```python
from build123d import *

# Parameters (mm, degrees)
SCHIZZO1_W                   = 120
SCHIZZO1_H                   = 40
ESTRUSIONE_ESTRUSIONE1_DEPTH = 3
SCHIZZO2_R                   = 2.5
TAGLIO_ESTRUSIONE1_DEPTH     = 3
SCHIZZO3_R                   = 2.5
TAGLIO_ESTRUSIONE2_DEPTH     = 3


with BuildPart() as part:
    # Schizzo1 → Estrusione-Estrusione1 (new body)
    with BuildSketch(Plane.XY):
        with Locations((60, -20)):
            Rectangle(SCHIZZO1_W, SCHIZZO1_H)
    extrude(amount=ESTRUSIONE_ESTRUSIONE1_DEPTH)

    # Schizzo2 → Taglio-Estrusione1 (cut)
    with BuildSketch(Plane.XY.offset(3)):
        with Locations((18, -20)):
            Circle(SCHIZZO2_R)
    extrude(amount=-TAGLIO_ESTRUSIONE1_DEPTH, mode=Mode.SUBTRACT)

    # Schizzo3 → Taglio-Estrusione2 (cut)
    with BuildSketch(Plane.XY.offset(3)):
        with Locations((100, -20)):
            Circle(SCHIZZO3_R)
    extrude(amount=-TAGLIO_ESTRUSIONE2_DEPTH, mode=Mode.SUBTRACT)


solid = part.part
```
Input: part model. Units: mm. Frame: model coordinates. Coordinates: 2 decimals unless noted, no trailing zeros. Loops run counter-clockwise (first coordinate to the right, second up) from the corner with the lowest first, then second, coordinate; pieces in that order, holes last. Notation, with made-up numbers: M 88,65.25 L 120,65.25 A18 ccw 120,77.25 Z; hole C 56,69 d6. An arc over 180 degrees is marked long. Use a Markdown table: item, result. Add a question column.
1) Line query: L1, parallel to Y at x = 100, z = 1.7; L2, parallel to X at y = -21, z = 1.35; L3, parallel to Y at x = 20, z = 0.9. Output: solid intervals per line, ascending. Write a range as from..to.
2) Section B-B, the plane x = 100. Return the cut outline in (y, z), plus the area to 3 significant figures.
3) Section A-A, the plane y = -20. Return the cut outline in (x, z).
4) Pin query (flat end, axial travel): P1, Ø6, axis at x = 103, y = -12.5, coming from the -Z side. Return the tip coordinate at first contact, or that it passes through.
5) Draft query along Y for faces 1 (the flat face through (59, 0, 1)), 2 (the cylindrical face through (101.34, -17.89, 1.52)), 3 (the cylindrical face through (15.5, -19.9, 1.5)), 4 (the flat face through (59, -20, 3)). Return one class per face: +Y half, -Y half, draft (parallel to the pull), parting line (faces both ways), or undercut.
Answer below:
| question | item | result |
|---|---|---|
| 1 | L1 | -40..-22.5, -17.5..0 |
| 1 | L2 | 0..15.71, 20.29..97.71, 102.29..120 |
| 1 | L3 | -40..-21.5, -18.5..0 |
| 2 | outline | M -40,0 L -22.5,0 L -22.5,3 L -40,3 Z; M -17.5,0 L 0,0 L 0,3 L -17.5,3 Z |
| 2 | area | 105 mm2 |
| 3 | outline | M 0,0 L 15.5,0 L 15.5,3 L 0,3 Z; M 20.5,0 L 97.5,0 L 97.5,3 L 20.5,3 Z; M 102.5,0 L 120,0 L 120,3 L 102.5,3 Z |
| 4 | P1 | z = 0 |
| 5 | face 1 | +Y half |
| 5 | face 2 | undercut |
| 5 | face 3 | undercut |
| 5 | face 4 | draft |
